For this review, use the dimensioned drawing (mm, ordinates from the lowest corner) and the shaded views. Give positions to 0.01 mm unless a question says otherwise; leave off trailing zeros. Loops run counter-clockwise (first coordinate to the right, second up) from the corner with the lowest first, then second, coordinate; pieces in that order, holes last. Notation, with made-up numbers: (47.5, 52.25) - (96.5, 52.25) arc R9 ccw to (96.5, 68.25) - close; hole circle Ø1 at (10.25, 21). An arc over 180 degrees is marked (long way). Write each question's results on one line, items separated by ' | '.
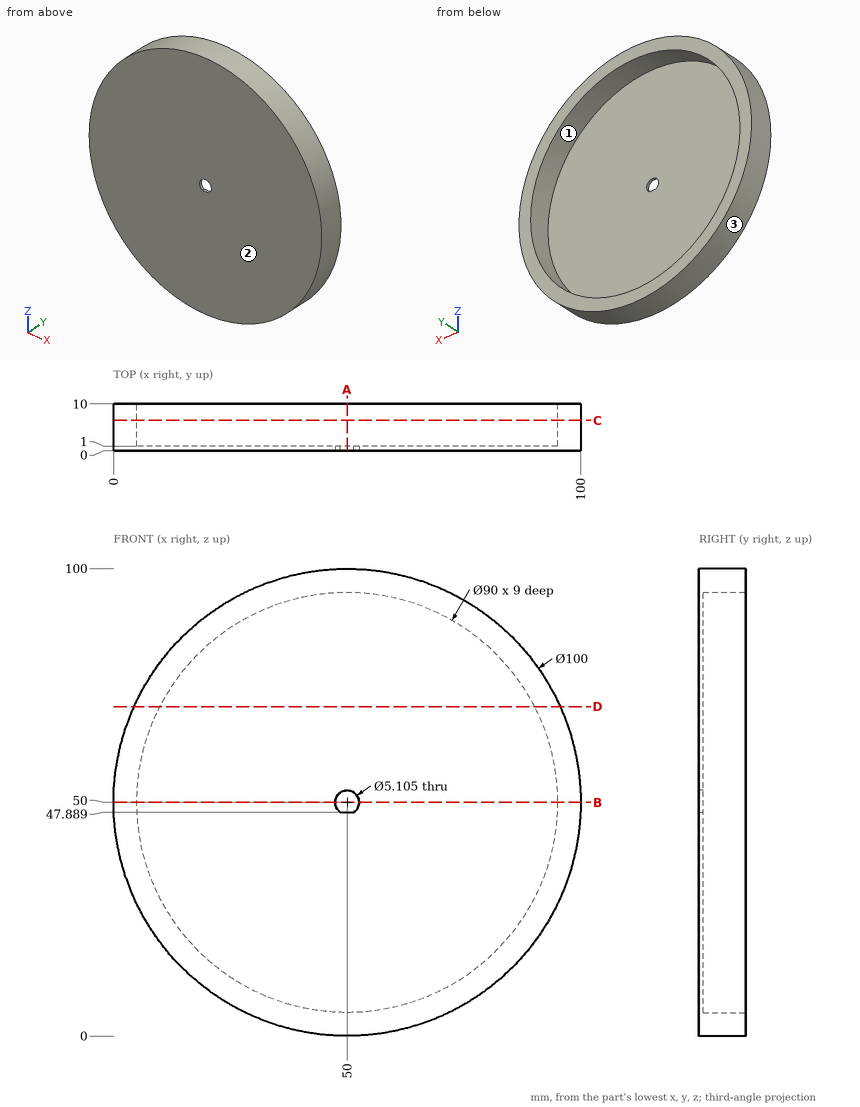
Item 1: We need section D-D on z = 70.5. Give the boundary of the cut face in (x, y) (1 decimal).
Output values:
outline: (4.4, 0) - (95.6, 0) - (95.6, 10) - (90.1, 10) - (90.1, 1) - (9.9, 1) - (9.9, 10) - (4.4, 10) - close
Item 2: We need section B-B on z = 50. Give the boundary of the cut face in (x, y).
Output values:
outline: (0, 0) - (47.45, 0) - (47.45, 1) - (5, 1) - (5, 10) - (0, 10) - close; (52.55, 0) - (100, 0) - (100, 10) - (95, 10) - (95, 1) - (52.55, 1) - close
Item 3: Clearance check with flat-ended pins moving along their axes: P1, Ø1, axis at y = 7.5, z = 12, coming from the +X side; P2, Ø2, axis at x = 18, y = 1.5, coming from the +Z side; P3, Ø1.5, axis at x = 89.5, y = 4.5, coming from the -Z side. State where each tip first meets the part, or that it passes through.
Output values:
P1: stops at x = 83.07 | P2: stops at z = 89.23 | P3: stops at z = 18.4
Item 4: We need section C-C on y = 6.5. Give the boundary of the cut face in (x, z), then the cut area to 3 significant figures.
Output values:
outline: circle Ø100 at (50, 50); hole circle Ø90 at (50, 50) | area: 1,490 mm²
Item 5: Draft analysis for pull direction Z (two halves, no side actions). For the marked faces 1, 2 and 3, state which applies: +Z half, -Z half, draft (parallel to the pull), parting line (faces both ways), or undercut.
Output values:
face 1: undercut | face 2: draft | face 3: parting line
Item 6: Wall thickness on probe 1 along Z at (x, y) = (50, 3.5); probe 2 along Y at (x, z) = (27, 27); probe 3 along X at (y, z) = (7.5, 47): over which ranges is each line inside the solid? List them lowest first.
Output values:
probe 1: z = 0 to 5, 95 to 100 | probe 2: y = 0 to 1 | probe 3: x = 0.09 to 5.1, 94.9 to 99.91
Item 7: We need section A-A on x = 50. Give the boundary of the cut face in (y, z).
Output values:
outline: (0, 0) - (10, 0) - (10, 5) - (1, 5) - (1, 47.89) - (0, 47.89) - close; (0, 52.55) - (1, 52.55) - (1, 95) - (10, 95) - (10, 100) - (0, 100) - close
